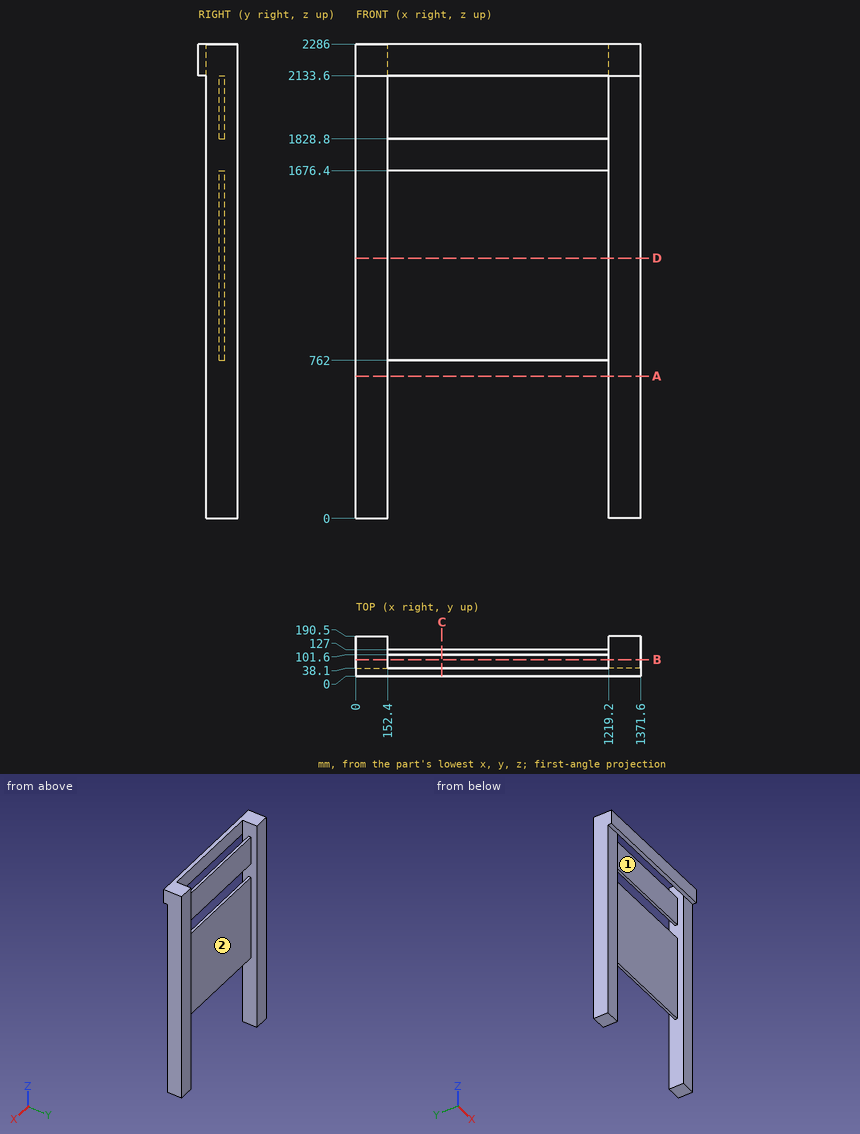
Can you work these out from the drawing? Everything is in mm from the part's minimum corner. A direction names the side the tool comes from. Give positions to 0.01 mm unless a question says otherwise; leave off trailing zeros. Loops run counter-clockwise (first coordinate to the right, second up) from the corner with the lowest first, then second, coordinate; pieces in that order, holes last. Notation, with made-up numbers: M -17,-22 L 17,-22 A22 ccw 17,6 Z; hole C 54,53 d4. An arc over 180 degrees is marked long. Put each result on its own line as item: value. Start each with the question number.
(1) Will these pins go through, and if not, where does the flat tip stop? pin 1 Ø10 at (x, z) = (718.5, 1517.5) entering from -Y; pin 2 Ø12.5 at (x, y) = (522.5, 114.5) entering from -Z; pin 3 Ø7.5 at (x, y) = (654.5, 119) entering from +Z.
(2) I want a section at D-D on z = 1254. Please give me the cut outline in (x, y).
(3) I want a section at B-B on y = 79. Please give me the cut outline in (x, z).
(4) I want a section at C-C on x = 414. Please give me the cut outline in (y, z), then the cut area to 3 significant figures.
(5) I want a section at A-A on z = 686. Please give me the cut outline in (x, y), then the cut area to 3 significant figures.
(6) I need wall thicknesses on line 1 along X through (y, z) = (69, 2017); line 2 along Z through (x, y) = (849, 115); line 3 along Y through (x, z) = (150, 1892.5). Which ranges of each line are inside material? Lowest first, please. Write a range as [from, to].
(7) For the marked faces 1 and 2, which set-ups out of +Z, -Z, +X, -X, +Y, -Y let a thin tool reach every point of the face, with its end or its side?
Answer block:
1. pin 1: y = 101.6
1. pin 2: z = 762
1. pin 3: z = 2133.6
2. outline: M 0,38.1 L 152.4,38.1 L 152.4,101.6 L 1219.2,101.6 L 1219.2,38.1 L 1371.6,38.1 L 1371.6,190.5 L 1219.2,190.5 L 1219.2,127 L 152.4,127 L 152.4,190.5 L 0,190.5 Z
3. outline: M 0,0 L 152.4,0 L 152.4,2286 L 0,2286 Z; M 1219.2,0 L 1371.6,0 L 1371.6,2286 L 1219.2,2286 Z
4. outline: M 0,2133.6 L 38.1,2133.6 L 38.1,2286 L 0,2286 Z; M 101.6,762 L 127,762 L 127,1676.4 L 101.6,1676.4 Z; M 101.6,1828.8 L 127,1828.8 L 127,2133.6 L 101.6,2133.6 Z
4. area: 36,800 mm^2
5. outline: M 0,38.1 L 152.4,38.1 L 152.4,190.5 L 0,190.5 Z; M 1219.2,38.1 L 1371.6,38.1 L 1371.6,190.5 L 1219.2,190.5 Z
5. area: 46,500 mm^2
6. line 1: [0, 152.4], [1219.2, 1371.6]
6. line 2: [762, 1676.4], [1828.8, 2133.6]
6. line 3: [38.1, 190.5]
7. face 1: +Z, -Z, -Y
7. face 2: +Z, -Z, +Y
